from build123d import *

# Parameters (mm, degrees)
BOSS_EXTRUDE1_DEPTH   = 7.5
CUT_EXTRUDE1_DEPTH    = 124.718430317
BOSS_EXTRUDE2_START   = 37.5
BOSS_EXTRUDE2_DEPTH   = 37.5
BOSS_EXTRUDE3_START   = 27.5
BOSS_EXTRUDE3_DEPTH   = 27.5
SKETCH4_R             = 7.5
BOSS_EXTRUDE4_DEPTH   = 15
MIRROR1_DEPTH         = 27.5
MIRROR1_2_DEPTH       = 7.5
MIRROR1_START         = 27.5
MIRROR1_3_OUTLINE_W   = 15
MIRROR1_3_OUTLINE_H   = 130
MIRROR1_3_OUTLINE_H_2 = 65
MIRROR1_3_DEPTH       = 14.9999999
MIRROR1_4_DEPTH       = 10
MIRROR1_START_2       = -120
MIRROR1_5_OUTLINE_R   = 7.5
MIRROR1_5_DEPTH       = 15
MIRROR1_START_3       = 105
MIRROR1_6_OUTLINE_R   = 7.5
MIRROR1_6_DEPTH       = 15


with BuildPart() as part:
    # Sketch1 → Boss-Extrude1 (new body)
    with BuildSketch(Plane(origin=(0, 0, 0), x_dir=(1, 0, 0), z_dir=(0, 1, 0))):
        with BuildLine():
            Line((43.979733232, 48.649668798), (105, 65))
            Line((105, 65), (105, 0))
            Line((105, 0), (0, 0))
            Line((0, 0), (0, 57))
            ThreePointArc((0, 57), (14.366743308, 55.159737914), (27.805817387, 49.757778482))
            ThreePointArc((27.805817387, 49.757778482), (35.800459234, 47.856282629), (43.979733232, 48.649668798))
        make_face()
    extrude(amount=BOSS_EXTRUDE1_DEPTH)

    # Sketch2 → Cut-Extrude1 (cut, through all)
    with BuildSketch(Plane(origin=(0, 7.5, 0), x_dir=(1, 0, 0), z_dir=(0, 1, 0))):
        with BuildLine():
            Line((0, 15), (0, 0))
            Line((0, 0), (15, 0))
            ThreePointArc((15, 0), (10.606601718, 10.606601718), (0, 15))
        make_face()
    extrude(amount=-CUT_EXTRUDE1_DEPTH, mode=Mode.SUBTRACT)

    # Sketch3 → Boss-Extrude2 (add)
    with BuildSketch(Plane(origin=(0, 0, 0), x_dir=(1, 0, 0), z_dir=(0, 1, 0)).offset(BOSS_EXTRUDE2_START)):
        with BuildLine():
            ThreePointArc((28.5, 0), (28.247747201, 3.783487555), (27.49545417, 7.5))
            ThreePointArc((27.49545417, 7.5), (17.298843892, 22.649503306), (0, 28.5))
            Line((0, 28.5), (0, 15))
            ThreePointArc((0, 15), (10.606601718, 10.606601718), (15, 0))
            Line((15, 0), (28.5, 0))
        make_face()
    extrude(amount=-BOSS_EXTRUDE2_DEPTH)

    # Sketch3<4> → Boss-Extrude3 (add)
    with BuildSketch(Plane(origin=(0, 0, 0), x_dir=(1, 0, 0), z_dir=(0, 1, 0)).offset(BOSS_EXTRUDE3_START)):
        with BuildLine():
            Line((105, 7.5), (27.49545417, 7.5))
            ThreePointArc((27.49545417, 7.5), (28.247747201, 3.783487555), (28.5, 0))
            Line((28.5, 0), (105, 0))
            Line((105, 0), (105, 7.5))
        make_face()
    extrude(amount=-BOSS_EXTRUDE3_DEPTH)

    # Sketch4 → Boss-Extrude4 (add)
    with BuildSketch(Plane(origin=(105, 0, 0), x_dir=(0, 0, -1), z_dir=(1, 0, 0))):
        with BuildLine():
            Line((0, 0), (65, 0))
            Line((65, 0), (65, 50))
            ThreePointArc((65, 50), (59.142135624, 64.142135624), (45, 70))
            Line((45, 70), (0, 70))
            Line((0, 70), (0, 0))
        make_face()
        with Locations((45, 50)):
            Circle(SKETCH4_R, mode=Mode.SUBTRACT)
    extrude(amount=BOSS_EXTRUDE4_DEPTH)

    # Mirror1: read off the stored shape, not the designer's step
    # Mirror1 outline → Mirror1 (add)
    with BuildSketch(Plane(origin=(0, 0, 0), x_dir=(1, 0, 0), z_dir=(0, 1, 0))):
        with BuildLine():
            Line((0, 15), (0, 28.5))
            ThreePointArc((0, 28.5), (-17.298843892, 22.649503306), (-27.49545417, 7.5))
            Line((-27.49545417, 7.5), (-105, 7.5))
            Line((-105, 7.5), (-105, 65))
            Line((-105, 65), (-120, 65))
            Line((-120, 65), (-120, -65))
            Line((-120, -65), (-105, -65))
            Line((-105, -65), (-105, -7.5))
            Line((-105, -7.5), (-27.49545417, -7.5))
            ThreePointArc((-27.49545417, -7.5), (0, -28.5), (27.49545417, -7.5))
            Line((27.49545417, -7.5), (105, -7.5))
            Line((105, -7.5), (105, -65))
            Line((105, -65), (120, -65))
            Line((120, -65), (120, 0))
            Line((120, 0), (15, 0))
            ThreePointArc((15, 0), (-10.606601718, -10.606601718), (0, 15))
        make_face()
    extrude(amount=MIRROR1_DEPTH)

    # Mirror1 2 outline → Mirror1 2 (add)
    with BuildSketch(Plane(origin=(0, 0, 0), x_dir=(1, 0, 0), z_dir=(0, 1, 0))):
        with BuildLine():
            ThreePointArc((0, 57), (-14.366743308, 55.159737914), (-27.805817387, 49.757778482))
            ThreePointArc((-27.805817387, 49.757778482), (-35.800459234, 47.856282629), (-43.979733232, 48.649668798))
            Line((-43.979733232, 48.649668798), (-105, 65))
            Line((-105, 65), (-105, 7.5))
            Line((-105, 7.5), (-27.49545417, 7.5))
            ThreePointArc((-27.49545417, 7.5), (-17.298843892, 22.649503306), (0, 28.5))
            Line((0, 28.5), (0, 57))
        make_face()
        with BuildLine():
            Line((105, -7.5), (27.49545417, -7.5))
            ThreePointArc((27.49545417, -7.5), (0, -28.5), (-27.49545417, -7.5))
            Line((-27.49545417, -7.5), (-105, -7.5))
            Line((-105, -7.5), (-105, -65))
            Line((-105, -65), (-43.979733232, -48.649668798))
            ThreePointArc((-43.979733232, -48.649668798), (-35.800459234, -47.856282629), (-27.805817387, -49.757778482))
            ThreePointArc((-27.805817387, -49.757778482), (0, -57), (27.805817387, -49.757778482))
            ThreePointArc((27.805817387, -49.757778482), (35.800459234, -47.856282629), (43.979733232, -48.649668798))
            Line((43.979733232, -48.649668798), (105, -65))
            Line((105, -65), (105, -7.5))
        make_face()
    extrude(amount=MIRROR1_2_DEPTH)

    # Mirror1 3 outline → Mirror1 3 (add)
    with BuildSketch(Plane(origin=(0, 0, 0), x_dir=(1, 0, 0), z_dir=(0, 1, 0)).offset(MIRROR1_START)):
        with Locations((-112.5, 0)):
            Rectangle(MIRROR1_3_OUTLINE_W, MIRROR1_3_OUTLINE_H)
        with Locations((112.5, -32.5)):
            Rectangle(MIRROR1_3_OUTLINE_W, MIRROR1_3_OUTLINE_H_2)
    extrude(amount=MIRROR1_3_DEPTH)

    # Mirror1 4 outline → Mirror1 4 (add)
    with BuildSketch(Plane(origin=(0, 0, 0), x_dir=(1, 0, 0), z_dir=(0, 1, 0)).offset(MIRROR1_START)):
        with BuildLine():
            Line((0, 15), (0, 28.5))
            ThreePointArc((0, 28.5), (-20.152543264, -20.152543264), (28.5, 0))
            Line((28.5, 0), (15, 0))
            ThreePointArc((15, 0), (-10.606601718, -10.606601718), (0, 15))
        make_face()
    extrude(amount=MIRROR1_4_DEPTH)

    # Mirror1 5 outline → Mirror1 5 (add)
    with BuildSketch(Plane.YZ.offset(MIRROR1_START_2)):
        with BuildLine():
            Line((7.5, -7.5), (7.5, -65))
            Line((7.5, -65), (50, -65))
            ThreePointArc((50, -65), (64.142135624, -59.142135624), (70, -45))
            Line((70, -45), (70, 45))
            ThreePointArc((70, 45), (64.142135624, 59.142135624), (50, 65))
            Line((50, 65), (7.5, 65))
            Line((7.5, 65), (7.5, 7.5))
            Line((7.5, 7.5), (27.5, 7.5))
            Line((27.5, 7.5), (27.5, -7.5))
            Line((27.5, -7.5), (7.5, -7.5))
        make_face()
        with Locations((50, -45)):
            Circle(MIRROR1_5_OUTLINE_R, mode=Mode.SUBTRACT)
        with Locations((50, 45)):
            Circle(MIRROR1_5_OUTLINE_R, mode=Mode.SUBTRACT)
    extrude(amount=MIRROR1_5_DEPTH)

    # Mirror1 6 outline → Mirror1 6 (add)
    with BuildSketch(Plane.YZ.offset(MIRROR1_START_3)):
        with BuildLine():
            Line((7.5, -7.5), (7.5, -65))
            Line((7.5, -65), (50, -65))
            ThreePointArc((50, -65), (64.142135624, -59.142135624), (70, -45))
            Line((70, -45), (70, 45))
            ThreePointArc((70, 45), (64.142135624, 59.142135624), (50, 65))
            Line((50, 65), (7.5, 65))
            Line((7.5, 65), (7.5, 7.5))
            Line((7.5, 7.5), (27.5, 7.5))
            Line((27.5, 7.5), (27.5, -7.5))
            Line((27.5, -7.5), (7.5, -7.5))
        make_face()
        with Locations((50, -45)):
            Circle(MIRROR1_6_OUTLINE_R, mode=Mode.SUBTRACT)
        with Locations((50, 45)):
            Circle(MIRROR1_6_OUTLINE_R, mode=Mode.SUBTRACT)
    extrude(amount=MIRROR1_6_DEPTH)

    # Mirror2: part across face


with BuildPart() as part_1:
    add(part.part)
    add(part.part.mirror(Plane(origin=(0, 0, 0), x_dir=(0, 0, 1), z_dir=(0, -1, 0))))


solid = part_1.part
Could you check a few things on this model? Use its own coordinates, in mm. A direction names the side the tool comes from. Round coordinates to 2 decimals unless told otherwise and drop trailing zeros. Loops run counter-clockwise (first coordinate to the right, second up) from the corner with the lowest first, then second, coordinate; pieces in that order, holes last. Notation, with made-up numbers: (44, 28) -> (50, 28) arc R20 ccw to (50, 45) -> close; hole circle Ø4 at (55, 32). An arc over 180 degrees is marked (long way). Use CSV: the item, a comma, the result in double quotes.
(1) If we mould it in two halves opening along Y, with no side actions, what happens to faces 1 (the cylindrical face through (35.685, 0.105, -47.864)), 2 (the cylindrical face through (112.395, 43.346, -48.461)), 3 (the flat face through (-1, 7.5, -37))? For each: +Y half, -Y half, draft (parallel to the pull), parting line (faces both ways), or undercut.
Return value:
face 1,"draft"
face 2,"undercut"
face 3,"+Y half"
(2) Suppose I cut it at B-B on y = 53.5. Write out the boundary of the cut face in (x, z).
Return value:
outline,"(-120, -64.69) -> (-105, -64.69) -> (-105, -51.63) -> (-120, -51.63) -> close; (-120, -38.37) -> (-105, -38.37) -> (-105, 38.37) -> (-120, 38.37) -> close; (-120, 51.63) -> (-105, 51.63) -> (-105, 64.69) -> (-120, 64.69) -> close; (105, -64.69) -> (120, -64.69) -> (120, -51.63) -> (105, -51.63) -> close; (105, -38.37) -> (120, -38.37) -> (120, 38.37) -> (105, 38.37) -> close; (105, 51.63) -> (120, 51.63) -> (120, 64.69) -> (105, 64.69) -> close"
(3) If I drill on probe 1 along Y at (x, z) = (115, 45); probe 2 along Z at (x, y) = (-111, -50); probe 3 along X at (y, z) = (56.5, -32), over which ranges is the centre line in solid material (lowest first)? Write a range as [from, to].
Return value:
probe 1,"y = [-70, -57.5], [-42.5, 42.5], [57.5, 70]"
probe 2,"z = [-65, -52.5], [-37.5, 37.5], [52.5, 65]"
probe 3,"x = [-120, -105], [105, 120]"
(4) Suppose I cut it at C-C on z = 10.5. Write out the boundary of the cut face in (x, y).
Return value:
outline,"(-120, -70) -> (-105, -70) -> (-105, -7.5) -> (-26.5, -7.5) -> (-26.5, -37.5) -> (-10.71, -37.5) -> (-10.71, 37.5) -> (-26.5, 37.5) -> (-26.5, 7.5) -> (-105, 7.5) -> (-105, 70) -> (-120, 70) -> close; (10.71, -37.5) -> (26.5, -37.5) -> (26.5, -7.5) -> (105, -7.5) -> (105, -70) -> (120, -70) -> (120, 70) -> (105, 70) -> (105, 7.5) -> (26.5, 7.5) -> (26.5, 37.5) -> (10.71, 37.5) -> close"
(5) Will these pins go through, and if not, where does the flat tip stop? pin 1 Ø8 at (x, y) = (44.5, 0.5) entering from -Z; pin 2 Ø6 at (x, y) = (-85.5, -15) entering from +Z; pin 3 Ø2 at (x, y) = (-0.5, -32.5) entering from -Z.
Return value:
pin 1,"stops at z = -49.86"
pin 2,"stops at z = 7.5"
pin 3,"stops at z = -28.5"
(6) For faces 4 (the flat face through (-1, -7.5, 36)), 5 (the flat face through (-1, -7.5, -37)), 6 (the flat face through (105, 39, 1)), which set-ups out of +Z, -Z, +X, -X, +Y, -Y let a thin tool reach every point of the face, with its end or its side?
Return value:
face 4,"+Z, -Y"
face 5,"-Z, -Y"
face 6,"+Y"
(7) Suppose I cut it at D-D on x = -85.5. Write out the boundary of the cut face in (y, z) (3 decimals), plus the area to 3 significant figures.
Return value:
outline,"(-27.5, -7.5) -> (-7.5, -7.5) -> (-7.5, -59.775) -> (7.5, -59.775) -> (7.5, -7.5) -> (27.5, -7.5) -> (27.5, 7.5) -> (7.5, 7.5) -> (7.5, 59.775) -> (-7.5, 59.775) -> (-7.5, 7.5) -> (-27.5, 7.5) -> close"
area,"2,390 mm²"
(8) Suppose I cut it at A-A on y = -1. Write out the boundary of the cut face in (x, z).
Return value:
outline,"(-120, -65) -> (-105, -65) -> (-43.98, -48.65) arc R25 cw to (-27.81, -49.76) arc R57 ccw to (27.81, -49.76) arc R25 cw to (43.98, -48.65) -> (105, -65) -> (120, -65) -> (120, 65) -> (105, 65) -> (43.98, 48.65) arc R25 cw to (27.81, 49.76) arc R57 ccw to (-27.81, 49.76) arc R25 cw to (-43.98, 48.65) -> (-105, 65) -> (-120, 65) -> close; hole circle Ø30 at (0, 0)"
